```python
from build123d import *

# Parameters (mm, degrees)
PAD002_DEPTH  = 105
SKETCH003_W   = 5.5
SKETCH003_H   = 15.5
PAD003_DEPTH  = 0.3
SKETCH010_W   = 7.3
SKETCH010_H   = 15
SKETCH010_W_2 = 11
POCKET_DEPTH  = 2


with BuildPart() as part:
    # Sketch002 → Pad002 (new body)
    with BuildSketch(Plane.XZ):
        Polygon((0, 35.75), (15.5, 35.75), (22.5, 28), (22.5, 0), (0, 0), align=None)
    extrude(amount=-PAD002_DEPTH)

    # Sketch003 (on Face2 of Pad002) → Pad003 (join)
    with BuildSketch(Plane(origin=(26.3189111748, 0, 23.7719197708), x_dir=(-0.670286258, 0, 0.7421026428), z_dir=(0.7421026428, 0, 0.670286258))):
        with Locations((11.25, -29.75)):
            Rectangle(SKETCH003_W, SKETCH003_H)
        with Locations((11.25, -49.75)):
            Rectangle(SKETCH003_W, SKETCH003_H)
        with Locations((11.25, -69.75)):
            Rectangle(SKETCH003_W, SKETCH003_H)
        with Locations((11.25, -89.75)):
            Rectangle(SKETCH003_W, SKETCH003_H)
    extrude(amount=PAD003_DEPTH)

    # Sketch010 (on Face3 of Pad002) → Pocket (cut)
    with BuildSketch(Plane(origin=(22.5, 0, 0), x_dir=(0, 0, 1), z_dir=(1, 0, 0))):
        with Locations((6.65, -29.5)):
            Rectangle(SKETCH010_W, SKETCH010_H)
        with Locations((6.65, -49.5)):
            Rectangle(SKETCH010_W, SKETCH010_H)
        with Locations((6.65, -69.5)):
            Rectangle(SKETCH010_W, SKETCH010_H)
        with Locations((6.65, -89.5)):
            Rectangle(SKETCH010_W, SKETCH010_H)
        with Locations((19, -29.5)):
            Rectangle(SKETCH010_W_2, SKETCH010_H)
        with Locations((19.0116166835, -49.4999966263)):
            Rectangle(SKETCH010_W_2, SKETCH010_H)
        with Locations((19.023233367, -69.4999932526)):
            Rectangle(SKETCH010_W_2, SKETCH010_H)
        with Locations((19.0348500505, -89.4999898789)):
            Rectangle(SKETCH010_W_2, SKETCH010_H)
    extrude(amount=-POCKET_DEPTH, mode=Mode.SUBTRACT)


solid = part.part
```
Verification items for the finished model (mm, model axes). A direction names the side the tool comes from. Coordinates: 2 decimals unless noted, no trailing zeros. Order: outer loops, then holes, each group sorted by start corner. A loop starts at its lowest first (then second) coordinate and runs counter-clockwise, first axis right, second up. Notation, with made-up numbers: (55.5, -32) - (72.5, -32) arc R18 ccw to (72.5, -15) - close; hole circle Ø11 at (-8, 18). An arc over 180 degrees is marked (long way). Return JSON: item names as keys, results as strings.
(1) Section check C-C, the plane y = 26. Record the cut outline in (x, z).
Filled sheet:
{"outline": "(0, 0) - (22.5, 0) - (22.5, 3) - (20.5, 3) - (20.5, 10.3) - (22.5, 10.3) - (22.5, 13.5) - (20.5, 13.5) - (20.5, 24.5) - (22.5, 24.5) - (22.5, 28) - (20.62, 30.08) - (20.84, 30.28) - (17.16, 34.36) - (16.93, 34.16) - (15.5, 35.75) - (0, 35.75) - close"}
(2) Mould release check, pull along Y, two halves, no side actions. Record for faces 1 (the flat face through (22, 22, 7)), 2 (the flat face through (19.03, 69.64, 32.29)): pulls with the +Y half, pulls with the -Y half, needs draft (parallel to the pull), parting line crosses it, or undercut.
Filled sheet:
{"face 1": "undercut", "face 2": "needs draft"}
(3) Access from +Z, -Z, +X, -X, +Y, -Y to the whole of each face (thin tool, end or side, straight path). Record for faces 3 (the flat face through (22, 97, 7)), 4 (the flat face through (11, 52, 0)).
Filled sheet:
{"face 3": "+X", "face 4": "-Z, +X, -X, +Y, -Y"}
(4) Go/stop test with flat-tipped pins: pin 1 (2 mm diameter, centred on y = 72, z = 8, fed in from +X); pin 2 (1.6 mm diameter, centred on x = 22, y = 93, fed in from +Z); pin 3 (1 mm diameter, centred on x = 21.5, y = 27, fed in from +Z). Record where each tip stops, or that it passes through.
Filled sheet:
{"pin 1": "stops at x = 20.5", "pin 2": "stops at z = 29.44", "pin 3": "stops at z = 29.66"}
(5) Section check B-B, the plane x = 19.5. Record the cut outline in (y, z), and give its area (3 significant figures).
Filled sheet:
{"outline": "(0, 0) - (105, 0) - (105, 31.32) - (97.5, 31.32) - (97.5, 31.77) - (82, 31.77) - (82, 31.32) - (77.5, 31.32) - (77.5, 31.77) - (62, 31.77) - (62, 31.32) - (57.5, 31.32) - (57.5, 31.77) - (42, 31.77) - (42, 31.32) - (37.5, 31.32) - (37.5, 31.77) - (22, 31.77) - (22, 31.32) - (0, 31.32) - close", "area": "3,320 mm^2"}
(6) Section check A-A, the plane y = 60. Record the cut outline in (x, z), and give its area (3 significant figures).
Filled sheet:
{"outline": "(0, 0) - (22.5, 0) - (22.5, 28) - (15.5, 35.75) - (0, 35.75) - close", "area": "777 mm^2"}
(7) Thickness scan on line 1 along Z through (x, y) = (21.25, 73.5); line 2 along X through (y, z) = (35, 8); line 3 along Z through (x, y) = (18.75, 23.5). Record the ranges inside material, lowest first.
Filled sheet:
{"line 1": "z = 0 to 3, 10.3 to 13.52, 24.52 to 29.38", "line 2": "x = 0 to 20.5", "line 3": "z = 0 to 32.6"}
